Input: part model. Units: mm. Frame: model coordinates. Face numbers are marked on the shaded views. Give positions to 0.01 mm unless a question says otherwise; leave off trailing zeros. Loops run counter-clockwise (first coordinate to the right, second up) from the corner with the lowest first, then second, coordinate; pieces in that order, holes last. Notation, with made-up numbers: (-24, 16) -> (6, 16) arc R29 ccw to (6, 41) -> close; hole circle Ø7 at (72, -12.5). An arc over 180 degrees is marked (long way). Use CSV: the item, a comma, the result in double quotes.
```python
from build123d import *

# Parameters (mm, degrees)
SKETCH_1_W          = 10
SKETCH_1_H          = 10
SKETCH_1_R          = 2
EXTRUDE_1_DEPTH     = 10
SKETCH_2_R          = 2
CUT_EXTRUDE_1_DEPTH = 10
SKETCH_3_R          = 2
CUT_EXTRUDE_2_DEPTH = 10


with BuildPart() as part:
    # 草图1 → 凸台-拉伸1 (new body)
    with BuildSketch(Plane(origin=(0, 0, 0), x_dir=(1, 0, 0), z_dir=(0, 1, 0))):
        Rectangle(SKETCH_1_W, SKETCH_1_H)
        with Locations(Location((0, 0, 0), (0, 0, 270))):
            Circle(SKETCH_1_R, mode=Mode.SUBTRACT)
    extrude(amount=EXTRUDE_1_DEPTH)

    # 草图2 → 切除-拉伸1 (cut)
    with BuildSketch(Plane.XY.offset(5)):
        with Locations((0, 5)):
            Circle(SKETCH_2_R)
    extrude(amount=-CUT_EXTRUDE_1_DEPTH, mode=Mode.SUBTRACT)

    # 草图3 → 切除-拉伸2 (cut)
    with BuildSketch(Plane(origin=(5, 0, 0), x_dir=(0, 0, -1), z_dir=(1, 0, 0))):
        with Locations((0, 5)):
            Circle(SKETCH_3_R)
    extrude(amount=-CUT_EXTRUDE_2_DEPTH, mode=Mode.SUBTRACT)


solid = part.part
```
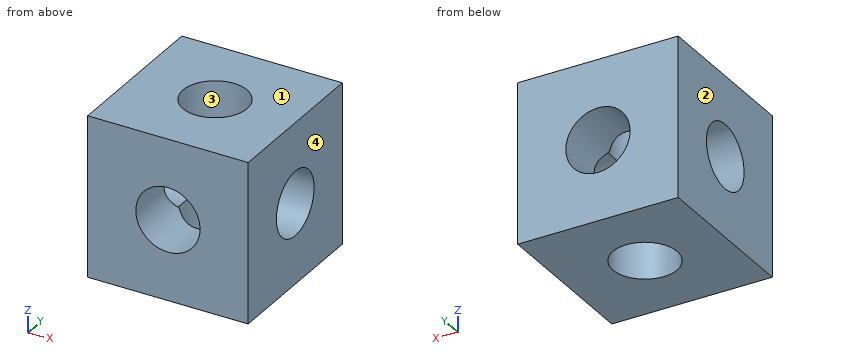
1) Section query A-A (x = 0). Return loops of the section in (y, z).
From the geometry:
outline,"(0, -5) -> (3, -5) -> (3, -2) -> (0, -2) -> close; (0, 2) -> (3, 2) -> (3, 5) -> (0, 5) -> close; (7, -5) -> (10, -5) -> (10, -2) -> (7, -2) -> close; (7, 2) -> (10, 2) -> (10, 5) -> (7, 5) -> close"
2) Section query B-B (y = 5). Return loops of the section in (x, z), then the cut area to 3 significant figures.
From the geometry:
outline,"(-5, -5) -> (-2, -5) -> (-2, -2) -> (-5, -2) -> close; (-5, 2) -> (-2, 2) -> (-2, 5) -> (-5, 5) -> close; (2, -5) -> (5, -5) -> (5, -2) -> (2, -2) -> close; (2, 2) -> (5, 2) -> (5, 5) -> (2, 5) -> close"
area,"36.0 mm^2"
3) Section query D-D (z = 3.75). Return loops of the section in (x, y).
From the geometry:
outline,"(-5, 0) -> (5, 0) -> (5, 10) -> (-5, 10) -> close; hole circle Ø4 at (0, 5)"
4) Mould query, pull axis X, two halves, no side actions, for the marked faces 1, 2, 3 and 4. Classes: pulls with the +X half, pulls with the -X half, needs draft (parallel to the pull), parting line crosses it, or undercut.
From the geometry:
face 1,"needs draft"
face 2,"pulls with the -X half"
face 3,"undercut"
face 4,"pulls with the +X half"
5) Section query C-C (x = 3.5). Return loops of the section in (y, z), then the cut area to 3 significant figures.
From the geometry:
outline,"(0, -5) -> (10, -5) -> (10, 5) -> (0, 5) -> close; hole circle Ø4 at (5, 0)"
area,"87.4 mm^2"
6) Ray query, line 1 (X direction, y = 5, z = 3.1); line 2 (Y direction, x = 0, z = 3.5). Return the intervals inside material, ascending.
From the geometry:
line 1,"x = -5 to -2, 2 to 5"
line 2,"y = 0 to 3, 7 to 10"
